Input: part model. Units: mm. Frame: model coordinates. Coordinates: 2 decimals unless noted, no trailing zeros. Write each loop counter-clockwise with the first axis right and the second up, starting at its lowest first coordinate (ties: lowest second). Pieces come first, ordered by that corner, then holes. Notation, with made-up numbers: (57.5, 54.5) - (64.5, 54.5) arc R8 ccw to (64.5, 58.5) - close; hole circle Ø1 at (32.5, 15). An arc over 180 degrees is marked (long way). Use a Markdown table: item, result. Add a question column.
Q1. Section query B-B (z = 44.45). Return the cut outline in (x, y), then the cut area to 3 significant figures.
Q2. Section query C-C (x = 0). Return the cut outline in (y, z), then the cut area to 3 significant figures.
Q3. Section query A-A (z = -50.8). Return the cut outline in (x, y).
Q4. Material intervals for probe 1 along Z at (x, y) = (0, -2.75); probe 2 along X at (y, z) = (-2.5, -50.8); probe 3 along X at (y, z) = (-5.75, 6), sorted ascending. Write a range as from..to.
Q5. Mould query, pull axis X, two halves, no side actions, for faces 1 (the face through (25.85, -3.13, -49.69)), 2 (the face through (-38.1, -3, 1)), 3 (the face through (-1, -3, -88.9)), 4 (the face through (1.47, -3.13, 4.05)). Classes: released by +X, released by -X, zero draft, split by the parting line, or undercut.
from build123d import *

# Parameters (mm, degrees)
SKETCH1_W           = 76.2
SKETCH1_H           = 177.8
SKETCH1_R           = 2.7305
SKETCH1_R_2         = 1.8288
BOSS_EXTRUDE1_DEPTH = 6.35


with BuildPart() as part:
    # Sketch1 → Boss-Extrude1 (new body)
    with BuildSketch(Plane(origin=(0, 0, 0), x_dir=(1, 0, 0), z_dir=(0, 1, 0))):
        Rectangle(SKETCH1_W, SKETCH1_H)
        with Locations((0, 69.85)):
            Circle(SKETCH1_R, mode=Mode.SUBTRACT)
        with Locations((0, 31.75)):
            Circle(SKETCH1_R, mode=Mode.SUBTRACT)
        with Locations((0, -6.35)):
            Circle(SKETCH1_R, mode=Mode.SUBTRACT)
        with Locations((0, -44.45)):
            Circle(SKETCH1_R, mode=Mode.SUBTRACT)
        with Locations((27.305, 50.8)):
            Circle(SKETCH1_R_2, mode=Mode.SUBTRACT)
        with Locations((27.305, 12.7)):
            Circle(SKETCH1_R_2, mode=Mode.SUBTRACT)
        with Locations((27.305, -25.4)):
            Circle(SKETCH1_R_2, mode=Mode.SUBTRACT)
        with Locations((-27.305, 12.7)):
            Circle(SKETCH1_R_2, mode=Mode.SUBTRACT)
        with Locations((-27.305, -25.4)):
            Circle(SKETCH1_R_2, mode=Mode.SUBTRACT)
        with Locations((-27.305, 50.8)):
            Circle(SKETCH1_R_2, mode=Mode.SUBTRACT)
    extrude(amount=-BOSS_EXTRUDE1_DEPTH)


solid = part.part
Values follow:
| question | item | result |
|---|---|---|
| 1 | outline | (-38.1, -6.35) - (-2.73, -6.35) - (-2.73, 0) - (-38.1, 0) - close; (2.73, -6.35) - (38.1, -6.35) - (38.1, 0) - (2.73, 0) - close |
| 1 | area | 449 mm2 |
| 2 | outline | (-6.35, -88.9) - (0, -88.9) - (0, -72.58) - (-6.35, -72.58) - close; (-6.35, -67.12) - (0, -67.12) - (0, -34.48) - (-6.35, -34.48) - close; (-6.35, -29.02) - (0, -29.02) - (0, 3.62) - (-6.35, 3.62) - close; (-6.35, 9.08) - (0, 9.08) - (0, 41.72) - (-6.35, 41.72) - close; (-6.35, 47.18) - (0, 47.18) - (0, 88.9) - (-6.35, 88.9) - close |
| 2 | area | 990 mm2 |
| 3 | outline | (-38.1, -6.35) - (-29.13, -6.35) - (-29.13, 0) - (-38.1, 0) - close; (-25.48, -6.35) - (25.48, -6.35) - (25.48, 0) - (-25.48, 0) - close; (29.13, -6.35) - (38.1, -6.35) - (38.1, 0) - (29.13, 0) - close |
| 4 | probe 1 | -88.9..-72.58, -67.12..-34.48, -29.02..3.62, 9.08..41.72, 47.18..88.9 |
| 4 | probe 2 | -38.1..-29.13, -25.48..25.48, 29.13..38.1 |
| 4 | probe 3 | -38.1..-2.71, 2.71..38.1 |
| 5 | face 1 | undercut |
| 5 | face 2 | released by -X |
| 5 | face 3 | zero draft |
| 5 | face 4 | undercut |
